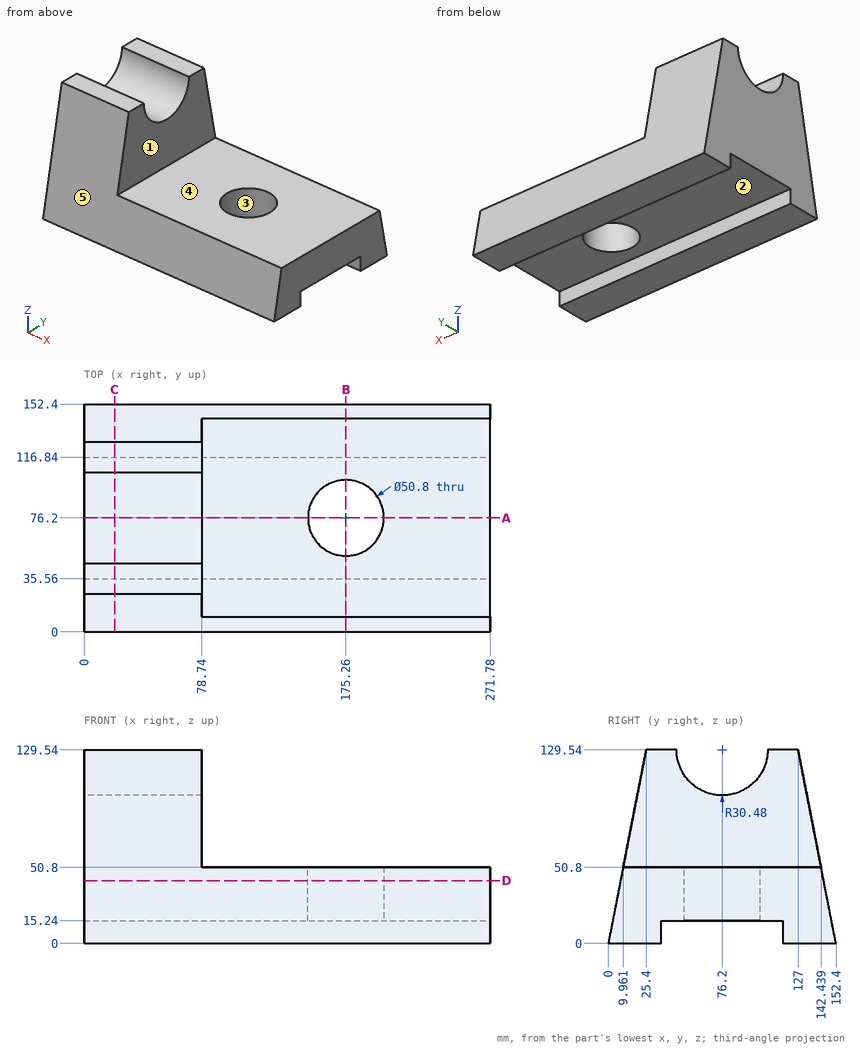
For this review, use the dimensioned drawing (mm, ordinates from the lowest corner) and the shaded views. A direction names the side the tool comes from. Round coordinates to 2 decimals unless told otherwise and drop trailing zeros. Write each loop counter-clockwise with the first axis right and the second up, starting at its lowest first coordinate (ties: lowest second). Pieces come first, ordered by that corner, then holes. Notation, with made-up numbers: M 3.5,0 L 45.5,0 A24 cw 45.5,22 Z; hole C 37,-33 d5. An arc over 180 degrees is marked long. Use CSV: the item, a comma, the result in double quotes. Start each with the question number.
(1) We need section B-B, the plane x = 175.26. State the section outline as (y, z) points.
(2) We need section A-A, the plane y = 76.2. State the section outline as (x, z) points.
(3) For line 1 along X through (y, z) = (76, 38); line 2 along Z through (x, y) = (124, 126); line 3 along X through (y, z) = (97, 72.5), list the stretches that pass through material, from the lowest coordinate up.
(4) Clearance check with flat-ended pins moving along their axes: P1, Ø12, axis at x = 116.5, y = 56, coming from the +Z side; P2, Ø12, axis at x = 89, z = 107, coming from the -Y side; P3, Ø7.5, axis at x = 170, z = 11, coming from the +Y side; P4, Ø1, axis at y = 81.5, z = 20, coming from the -X side. State where each tip first meets the part, or that it passes through.
(5) Tool access review of the marked faces 4 and 5: name each direction out of +Z, -Z, +X, -X, +Y, -Y from which nothing blocks a thin tool from reaching the whole face with its end or side.
(6) We need section D-D, the plane z = 42. State the section outline as (x, y) points (1 decimal).
(7) The part is to be moulded in two halves that separate along X. For the marked faces 1, 2 and 3, say which applies: +X half, -X half, draft (parallel to the pull), parting line (faces both ways), or undercut.
(8) We need section C-C, the plane x = 20.5. State the section outline as (y, z) points, then the cut area to 3 significant figures.
Findings:
1,outline,"M 0,0 L 35.56,0 L 35.56,15.24 L 50.8,15.24 L 50.8,50.8 L 9.96,50.8 Z; M 101.6,15.24 L 116.84,15.24 L 116.84,0 L 152.4,0 L 142.44,50.8 L 101.6,50.8 Z"
2,outline,"M 0,15.24 L 149.86,15.24 L 149.86,50.8 L 78.74,50.8 L 78.74,99.06 L 0,99.06 Z; M 200.66,15.24 L 271.78,15.24 L 271.78,50.8 L 200.66,50.8 Z"
3,line 1,"0 to 149.86, 200.66 to 271.78"
3,line 2,"0 to 50.8"
3,line 3,"0 to 78.74"
4,P1,"z = 50.8"
4,P2,"through"
4,P3,"y = 150.98"
4,P4,"x = 0"
5,face 4,"+Z, +X, +Y, -Y"
5,face 5,"+Z, +X, -X, -Y"
6,outline,"M 0,8.2 L 271.8,8.2 L 271.8,144.2 L 0,144.2 Z; hole C 175.3,76.2 d50.8"
7,face 1,"+X half"
7,face 2,"draft"
7,face 3,"undercut"
8,outline,"M 0,0 L 35.56,0 L 35.56,15.24 L 116.84,15.24 L 116.84,0 L 152.4,0 L 127,129.54 L 106.68,129.54 A30.48 cw 45.72,129.54 L 25.4,129.54 Z"
8,area,"13,800 mm^2"
